Input: part model. Units: mm. Frame: model coordinates. A direction names the side the tool comes from. Round coordinates to 2 decimals unless told otherwise and drop trailing zeros. Write each loop counter-clockwise with the first axis right and the second up, starting at its lowest first coordinate (ties: lowest second). Pieces come first, ordered by that corner, then holes. Notation, with made-up numbers: M 32.5,-4.75 L 39.5,-4.75 A21 cw 39.5,26.25 Z; hole C 13.5,70.5 d7. An arc over 180 degrees is marked long. Write each question's results on one line, items separated by ' | '. Start each with the question number.
```python
from build123d import *

# Parameters (mm, degrees)
F0_W      = 15.7988
F0_H      = 15.7988
F1_DEPTH  = 4.7879
F2_R      = 2.454504
F6_DEPTH  = 1.778
F3_R      = 2.4511
F7_DEPTH  = 1.778
F4_R      = 2.4511
F8_DEPTH  = 1.778
F5_R      = 2.4511
F9_DEPTH  = 1.778
F10_W     = 14.667356
F10_H     = 14.690364
F13_DEPTH = 8.3312
F11_R     = 3.2004
F14_DEPTH = 8.3312
F12_R     = 2.794
F15_DEPTH = 8.3312


with BuildPart() as f1:
    # F0 (on Top) → F1 (new body, symmetric)
    with BuildSketch(Plane.XY):
        Rectangle(F0_W, F0_H)
    extrude(amount=F1_DEPTH, both=True)

    # F2 (on face) → F6 (join)
    with BuildSketch(Plane.XY.offset(4.7879)):
        with Locations((-3.978046, 3.971696)):
            Circle(F2_R)
    extrude(amount=F6_DEPTH)

    # F3 (on face) → F7 (join)
    with BuildSketch(Plane.XY.offset(4.7879)):
        with Locations((3.9751, 3.9751)):
            Circle(F3_R)
    extrude(amount=F7_DEPTH)

    # F4 (on face) → F8 (join)
    with BuildSketch(Plane.XY.offset(4.7879)):
        with Locations((-3.9751, -3.9751)):
            Circle(F4_R)
    extrude(amount=F8_DEPTH)

    # F5 (on face) → F9 (join)
    with BuildSketch(Plane.XY.offset(4.7879)):
        with Locations((3.9751, -3.9751)):
            Circle(F5_R)
    extrude(amount=F9_DEPTH)

    # F10 (on face) → F13 (cut)
    with BuildSketch(Plane(origin=(0, 0, -4.7879), x_dir=(1, 0, 0), z_dir=(0, 0, -1))):
        Rectangle(F10_W, F10_H)
    extrude(amount=-F13_DEPTH, mode=Mode.SUBTRACT)

    # F11 (on face) → F14 (join)
    with BuildSketch(Plane(origin=(0, 0, -4.7879), x_dir=(1, 0, 0), z_dir=(0, 0, -1))):
        Circle(F11_R)
    extrude(amount=-F14_DEPTH)

    # F12 (on face) → F15 (cut)
    with BuildSketch(Plane(origin=(0, 0, -4.7879), x_dir=(1, 0, 0), z_dir=(0, 0, -1))):
        Circle(F12_R)
    extrude(amount=-F15_DEPTH, mode=Mode.SUBTRACT)


solid = f1.part
```
1. Cut plane A-A on z = -4. Output: boundary loops of the cut face in (x, y).
2. Line query: L1, parallel to X at y = 0, z = -0.25; L2, parallel to Y at x = 0, z = 0; L3, parallel to Y at x = -6, z = -3. Output: solid intervals per line, ascending. Write a range as from..to.
3. Cut plane C-C on y = 0. Output: boundary loops of the cut face in (x, z).
4. Draft query along X for faces 1 (the face through (0, 7.899, 0)), 2 (the face through (0, 7.345, -1)), 3 (the face through (7.899, 0, 0)). Return one class per face: +X half, -X half, draft (parallel to the pull), parting line (faces both ways), or undercut.
5. Contact query for a flat-ended pin moving along its axis: P1, Ø5, axis at x = 0, y = 0, coming from the -Z side. Output: stop coordinate, or through.
6. Cut plane D-D on z = 5. Output: boundary loops of the cut face in (x, y), and give its area (4 significant figures).
7. Access query for faces 4 (the face through (-3.4, -0.1, 3.543)), 5 (the face through (0, 3, -4.788)), 6 (the face through (-6.43, 4.08, 5.66)). Directions: +Z, -Z, +X, -X, +Y, -Y. A direction counts if a zero-diameter tool reaches every point of the face in a straight line with its end or side. Return the directions, or none.
8. Cut plane B-B on x = 0. Output: boundary loops of the cut face in (y, z), and give its area (3 significant figures).
Answers follow:
1) outline: M -7.9,-7.9 L 7.9,-7.9 L 7.9,7.9 L -7.9,7.9 Z; C 0,0 d6.4; hole M -7.33,-7.35 L 7.33,-7.35 L 7.33,7.35 L -7.33,7.35 Z; hole C 0,0 d5.59
2) L1: x = -7.9..-7.33, -3.2..-2.79, 2.79..3.2, 7.33..7.9 | L2: y = -7.9..-7.35, -3.2..-2.79, 2.79..3.2, 7.35..7.9 | L3: y = -7.9..-7.35, 7.35..7.9
3) outline: M -7.9,-4.79 L -7.33,-4.79 L -7.33,3.54 L -3.2,3.54 L -3.2,-4.79 L -2.79,-4.79 L -2.79,3.54 L 2.79,3.54 L 2.79,-4.79 L 3.2,-4.79 L 3.2,3.54 L 7.33,3.54 L 7.33,-4.79 L 7.9,-4.79 L 7.9,4.79 L -7.9,4.79 Z
4) face 1: draft | face 2: undercut | face 3: +X half
5) P1: stops at z = 3.54
6) outline: C -3.98,-3.98 d4.9; C -3.98,3.97 d4.91; C 3.98,-3.98 d4.9; C 3.98,3.98 d4.9 | area: 75.55 mm2
7) face 4: -Z | face 5: -Z, +X, -X, +Y, -Y | face 6: +Z
8) outline: M -7.9,-4.79 L -7.35,-4.79 L -7.35,3.54 L -3.2,3.54 L -3.2,-4.79 L -2.79,-4.79 L -2.79,3.54 L 2.79,3.54 L 2.79,-4.79 L 3.2,-4.79 L 3.2,3.54 L 7.35,3.54 L 7.35,-4.79 L 7.9,-4.79 L 7.9,4.79 L -7.9,4.79 Z | area: 35.7 mm2
